```python
from build123d import *

# Parameters (mm, degrees)
F0_W     = 25.4
F0_H     = 50.8
F0_W_2   = 19.05
F0_H_2   = 44.45
F1_DEPTH = 469.9
F2_R     = 14.2875
F2_R_2   = 3.175
F3_DEPTH = 25.4


with BuildPart() as f1:
    # F0 (on Front) → F1 (new body)
    with BuildSketch(Plane.XZ):
        Rectangle(F0_W, F0_H)
        Rectangle(F0_W_2, F0_H_2, mode=Mode.SUBTRACT)
    extrude(amount=F1_DEPTH)

    # F2 (on face) → F3 (cut)
    with BuildSketch(Plane.YZ.offset(12.7)):
        with Locations((-317.5, 0)):
            Circle(F2_R)
        with Locations((-139.7, -6.35)):
            Circle(F2_R_2)
    extrude(amount=-F3_DEPTH, mode=Mode.SUBTRACT)


solid = f1.part
```
Input: part model. Units: mm. Frame: model coordinates. A direction names the side the tool comes from. Coordinates: 2 decimals unless noted, no trailing zeros. Write each loop counter-clockwise with the first axis right and the second up, starting at its lowest first coordinate (ties: lowest second). Pieces come first, ordered by that corner, then holes.
1) Section B-B on x = 4.75. Output: boundary loops of the cut face in (y, z) (3 decimals).
2) Material intervals for line 1 along X through (y, z) = (-38, -18) (3 decimals); line 2 along Y through (x, z) = (11, 1); line 3 along Z through (x, y) = (-8.25, -93.5) (3 decimals), sorted ascending.
3) Set-up query: faces 4 (the flat face through (-9.525, -232, 0)), 5 (the flat face through (0, -232, -25.4)). Return all of +Z, -Z, +X, -X, +Y, -Y with unobstructed straight access to the full face (end or side cutting, diameter ignored); none if empty.
4) Mould query, pull axis Y, two halves, no side actions, for faces 1 (the cylindrical face through (11.135, -331.774, 0.628)), 2 (the flat face through (9.525, -232, 0)), 3 (the flat face through (-10, 0, -2)). Classes: pulls with the +Y half, pulls with the -Y half, needs draft (parallel to the pull), parting line crosses it, or undercut.
5) Section A-A on y = -354. Output: boundary loops of the cut face in (x, z) (3 decimals).
Check result:
1. outline: (-469.9, -25.4) - (0, -25.4) - (0, -22.225) - (-469.9, -22.225) - close; (-469.9, 22.225) - (0, 22.225) - (0, 25.4) - (-469.9, 25.4) - close
2. line 1: x = -12.7 to -9.525, 9.525 to 12.7
2. line 2: y = -469.9 to -331.75, -303.25 to 0
2. line 3: z = -25.4 to -22.225, 22.225 to 25.4
3. face 4: +Y, -Y
3. face 5: -Z, +X, -X, +Y, -Y
4. face 1: undercut
4. face 2: needs draft
4. face 3: pulls with the +Y half
5. outline: (-12.7, -25.4) - (12.7, -25.4) - (12.7, 25.4) - (-12.7, 25.4) - close; hole (-9.525, -22.225) - (9.525, -22.225) - (9.525, 22.225) - (-9.525, 22.225) - close
